from build123d import *

# Parameters (mm, degrees)
BOSS_EXTRUDE1_DEPTH = 50
SKETCH2_R           = 1.6
CUT_EXTRUDE1_DEPTH  = 50
SKETCH3_R           = 8.1
CUT_EXTRUDE2_DEPTH  = 50


with BuildPart() as part:
    # Sketch1 → Boss-Extrude1 (new body)
    with BuildSketch(Plane.XY):
        with BuildLine():
            Line((0, 35), (0, 2))
            ThreePointArc((0, 2), (0.585786438, 0.585786438), (2, 0))
            Line((2, 0), (16, 0))
            Line((16, 0), (16, 2))
            Line((16, 2), (3, 2))
            ThreePointArc((3, 2), (2.292893219, 2.292893219), (2, 3))
            Line((2, 3), (2, 35))
            Line((2, 35), (0, 35))
        make_face()
    extrude(amount=BOSS_EXTRUDE1_DEPTH)

    # Sketch2 → Cut-Extrude1 (cut)
    with BuildSketch(Plane(origin=(0, 2, 0), x_dir=(1, 0, 0), z_dir=(0, 1, 0))):
        with Locations(Location((9.5, -18.5, 0), (0, 0, 270))):
            Circle(SKETCH2_R)
        with Locations(Location((9.5, -31.5, 0), (0, 0, 270))):
            Circle(SKETCH2_R)
    extrude(amount=-CUT_EXTRUDE1_DEPTH, mode=Mode.SUBTRACT)

    # Sketch3 → Cut-Extrude2 (cut)
    with BuildSketch(Plane(origin=(2, 0, 0), x_dir=(0, 0, -1), z_dir=(1, 0, 0))):
        with Locations(Location((-12, 23, 0), (0, 0, 90))):
            Circle(SKETCH3_R)
        with Locations(Location((-38, 23, 0), (0, 0, 90))):
            Circle(SKETCH3_R)
        with BuildLine():
            ThreePointArc((-50, 23), (-46.485281374, 31.485281374), (-38, 35))
            Line((-38, 35), (-50, 35))
            Line((-50, 35), (-50, 23))
        make_face()
        with BuildLine():
            ThreePointArc((-22.2198998, 29.289169108), (-17.8536301, 33.475448184), (-12, 35))
            Line((-12, 35), (-38, 35))
            ThreePointArc((-38, 35), (-32.1463699, 33.475448184), (-27.7801002, 29.289169108))
            ThreePointArc((-27.7801002, 29.289169108), (-25, 27.735662478), (-22.2198998, 29.289169108))
        make_face()
        with BuildLine():
            Line((0, 35), (-12, 35))
            ThreePointArc((-12, 35), (-3.514718626, 31.485281374), (0, 23))
            Line((0, 23), (0, 35))
        make_face()
    extrude(amount=-CUT_EXTRUDE2_DEPTH, mode=Mode.SUBTRACT)


solid = part.part
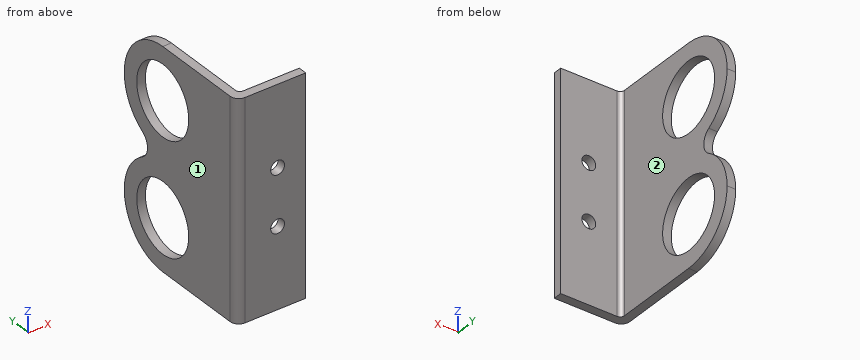
Source: CAD feature listing. Evaluate the final solid. Frame: model axes, mm. Face numbers are marked on the shaded views. A direction names the side the tool comes from. Round coordinates to 2 decimals unless told otherwise and drop trailing zeros. Loops run counter-clockwise (first coordinate to the right, second up) from the corner with the lowest first, then second, coordinate; pieces in that order, holes last.
Q1. Section C-C, the plane x = 5.75. Return loops of the section in (y, z).
Q2. Section D-D, the plane z = 31.5. Return loops of the section in (x, y), plus the area to 3 significant figures.
Q3. Access query for the marked faces 1 and 2. Directions: +Z, -Z, +X, -X, +Y, -Y. A direction counts if a zero-diameter tool reaches every point of the face in a straight line with its end or side. Return the directions, or none.
Q4. Ray query, line 1 (Z direction, x = 1.3, y = 23); line 2 (X direction, y = 5, z = 19). Return the intervals inside material, ascending.
Q5. Section B-B, the plane y = 32. Return loops of the section in (x, z), plus the area to 3 significant figures.
Q6. Section A-A, the plane z = 10. Return loops of the section in (x, y), plus the area to 3 significant figures.
Q7. First-contact query: P1, Ø4, axis at x = 1.5, y = 24.5, coming from the -Z side; P2, Ø1.5, axis at y = 12.5, z = 37, coming from the +X side; P3, Ø8, axis at x = 4.5, z = 21.5, coming from the +Y side (3 decimals); P4, Ø5, axis at x = 9.5, z = 31.5, coming from the +Y side. Flat tips, straight axial feed; report the tip coordinate or a pass-through.
Solutions:
1. outline: (0, 0) - (2, 0) - (2, 50) - (0, 50) - close
2. outline: (0, 2) arc R2 ccw to (2, 0) - (7.9, 0) - (7.9, 2) - (3, 2) arc R1 cw to (2, 3) - (2, 18.17) - (0, 18.17) - close; (0, 27.83) - (2, 27.83) - (2, 33.09) - (0, 33.09) - close; (11.1, 0) - (16, 0) - (16, 2) - (11.1, 2) - close
2. area: 67.8 mm2
3. face 1: +Z, -Z, -X, +Y, -Y
3. face 2: +Z, -Z, +X, +Y
4. line 1: z = 0 to 3.9, 20.1 to 29.9, 46.1 to 50
4. line 2: x = 0 to 2
5. outline: (0, 4.06) - (2, 4.06) - (2, 19.94) - (0, 19.94) - close; (0, 30.06) - (2, 30.06) - (2, 45.94) - (0, 45.94) - close
5. area: 63.5 mm2
6. outline: (0, 2) arc R2 ccw to (2, 0) - (16, 0) - (16, 2) - (3, 2) arc R1 cw to (2, 3) - (2, 15.15) - (0, 15.15) - close; (0, 30.85) - (2, 30.85) - (2, 34.83) - (0, 34.83) - close
6. area: 65.6 mm2
7. P1: stops at z = 0
7. P2: stops at x = 2
7. P3: stops at y = 33.165
7. P4: stops at y = 2
